```python
from build123d import *

# Parameters (mm, degrees)
SKETCH_1_R      = 2.08
SKETCH_1_R_2    = 8.75
SKETCH_1_R_3    = 1.5
EXTRUDE_2_DEPTH = 2


with BuildPart() as part:
    # 草图1 → 凸台-拉伸2 (new body)
    with BuildSketch(Plane.XY):
        with BuildLine():
            Line((25.488968202, 12.5), (30, 12.5))
            Line((30, 12.5), (30, 15.5))
            Line((30, 15.5), (37, 15.5))
            Line((37, 15.5), (37, 12.5))
            Line((37, 12.5), (41, 12.5))
            Line((41, 12.5), (41, 9.25))
            Line((41, 9.25), (44, 9.25))
            Line((44, 9.25), (44, 4.25))
            Line((44, 4.25), (41, 4.25))
            Line((41, 4.25), (41, 1.5))
            Line((41, 1.5), (38.5, 1.5))
            Line((38.5, 1.5), (38.5, 3))
            Line((38.5, 3), (35.9, 3))
            Line((35.9, 3), (35.9, 1.5))
            Line((35.9, 1.5), (32.9, 1.5))
            Line((32.9, 1.5), (32.9, -1.5))
            Line((32.9, -1.5), (35.9, -1.5))
            Line((35.9, -1.5), (35.9, -3))
            Line((35.9, -3), (38.5, -3))
            Line((38.5, -3), (38.5, -1.5))
            Line((38.5, -1.5), (41, -1.5))
            Line((41, -1.5), (41, -4.25))
            Line((41, -4.25), (44, -4.25))
            Line((44, -4.25), (44, -9.25))
            Line((44, -9.25), (41, -9.25))
            Line((41, -9.25), (41, -12.5))
            Line((41, -12.5), (37, -12.5))
            Line((37, -12.5), (37, -15.5))
            Line((37, -15.5), (30, -15.5))
            Line((30, -15.5), (30, -12.5))
            ThreePointArc((30, -12.5), (28.87224205, -11.37224205), (27.744484101, -12.5))
            Line((27.744484101, -12.5), (25.488968202, -12.5))
            ThreePointArc((25.488968202, -12.5), (0, -23.05787632), (-25.488968202, -12.5))
            Line((-25.488968202, -12.5), (-30, -12.5))
            Line((-30, -12.5), (-30, -15.5))
            Line((-30, -15.5), (-37, -15.5))
            Line((-37, -15.5), (-37, -12.5))
            Line((-37, -12.5), (-41, -12.5))
            Line((-41, -12.5), (-41, -9.25))
            Line((-41, -9.25), (-44, -9.25))
            Line((-44, -9.25), (-44, -4.25))
            Line((-44, -4.25), (-41, -4.25))
            Line((-41, -4.25), (-41, -1.5))
            Line((-41, -1.5), (-38.5, -1.5))
            Line((-38.5, -1.5), (-38.5, -3))
            Line((-38.5, -3), (-35.9, -3))
            Line((-35.9, -3), (-35.9, -1.5))
            Line((-35.9, -1.5), (-32.9, -1.5))
            Line((-32.9, -1.5), (-32.9, 1.5))
            Line((-32.9, 1.5), (-35.9, 1.5))
            Line((-35.9, 1.5), (-35.9, 3))
            Line((-35.9, 3), (-38.5, 3))
            Line((-38.5, 3), (-38.5, 1.5))
            Line((-38.5, 1.5), (-41, 1.5))
            Line((-41, 1.5), (-41, 4.25))
            Line((-41, 4.25), (-44, 4.25))
            Line((-44, 4.25), (-44, 9.25))
            Line((-44, 9.25), (-41, 9.25))
            Line((-41, 9.25), (-41, 12.5))
            Line((-41, 12.5), (-37, 12.5))
            Line((-37, 12.5), (-37, 15.5))
            Line((-37, 15.5), (-30, 15.5))
            Line((-30, 15.5), (-30, 12.5))
            Line((-30, 12.5), (-25.488968202, 12.5))
            ThreePointArc((-25.488968202, 12.5), (0, 23.05787632), (25.488968202, 12.5))
        make_face()
        with Locations((0, 13.53)):
            Circle(SKETCH_1_R, mode=Mode.SUBTRACT)
        with Locations((11.717323713, -6.765)):
            Circle(SKETCH_1_R, mode=Mode.SUBTRACT)
        with Locations((-11.717323713, -6.765)):
            Circle(SKETCH_1_R, mode=Mode.SUBTRACT)
        Circle(SKETCH_1_R_2, mode=Mode.SUBTRACT)
        with Locations((-12.990381057, 7.5)):
            Circle(SKETCH_1_R_3, mode=Mode.SUBTRACT)
        with Locations((12.990381057, 7.5)):
            Circle(SKETCH_1_R_3, mode=Mode.SUBTRACT)
        with Locations((0, -15)):
            Circle(SKETCH_1_R_3, mode=Mode.SUBTRACT)
    extrude(amount=EXTRUDE_2_DEPTH)


solid = part.part
```
Input: part model. Units: mm. Frame: model coordinates. A direction names the side the tool comes from. Give positions to 0.01 mm unless a question says otherwise; leave off trailing zeros. Loops run counter-clockwise (first coordinate to the right, second up) from the corner with the lowest first, then second, coordinate; pieces in that order, holes last.
1) Section query C-C on x = 10.5. Return the cut outline in (y, z), and give its area (3 significant figures).
A:
outline: (-21.49, 0) - (-8.45, 0) - (-8.45, 2) - (-21.49, 2) - close; (-5.08, 0) - (21.49, 0) - (21.49, 2) - (-5.08, 2) - close
area: 79.2 mm2
2) Reachability of faces 4 (the flat face through (30, -14, 1)), 5 (the flat face through (-43, -4.25, 1)), 6 (the flat face through (39, -12.5, 1)), 7 (the flat face through (-33, -15.5, 1)), 8 (the flat face through (43, 4.25, 1)) from +Z, -Z, +X, -X, +Y, -Y: full face, straight path, thin tool, end or side. Return the list, or none.
A:
face 4: +Z, -Z, -Y
face 5: +Z, -Z, -X
face 6: +Z, -Z, +X, -Y
face 7: +Z, -Z, -X, -Y
face 8: +Z, -Z, +X
3) Section query A-A on x = 0. Return the cut outline in (y, z), and give its area (3 significant figures).
A:
outline: (-23.06, 0) - (-16.5, 0) - (-16.5, 2) - (-23.06, 2) - close; (-13.5, 0) - (-8.75, 0) - (-8.75, 2) - (-13.5, 2) - close; (8.75, 0) - (11.45, 0) - (11.45, 2) - (8.75, 2) - close; (15.61, 0) - (23.06, 0) - (23.06, 2) - (15.61, 2) - close
area: 42.9 mm2
4) Line query: L1, parallel to Y at x = 0, z = 1.55; L2, parallel to Y at x = 36.5, z = 1.5; L3, parallel to Y at x = -40, z = 1.55. Output: solid intervals per line, ascending.
A:
L1: y = -23.06 to -16.5, -13.5 to -8.75, 8.75 to 11.45, 15.61 to 23.06
L2: y = -15.5 to -3, 3 to 15.5
L3: y = -12.5 to -1.5, 1.5 to 12.5
5) Section query D-D on y = 13.53. Return the cut outline in (x, z).
A:
outline: (-37, 0) - (-30, 0) - (-30, 2) - (-37, 2) - close; (-24.42, 0) - (-2.08, 0) - (-2.08, 2) - (-24.42, 2) - close; (2.08, 0) - (24.42, 0) - (24.42, 2) - (2.08, 2) - close; (30, 0) - (37, 0) - (37, 2) - (30, 2) - close
6) Mould query, pull axis Y, two halves, no side actions, for faces 1 (the flat face through (38.5, -2, 1)), 2 (the flat face through (44, 7, 1)), 3 (the flat face through (28, 12.5, 1)). Classes: released by +Y, released by -Y, zero draft, split by the parting line, or undercut.
A:
face 1: undercut
face 2: zero draft
face 3: released by +Y
7) Section query B-B on y = 0. Return the cut outline in (x, z).
A:
outline: (-32.9, 0) - (-8.75, 0) - (-8.75, 2) - (-32.9, 2) - close; (8.75, 0) - (32.9, 0) - (32.9, 2) - (8.75, 2) - close
8) Contact query for flat-ended pins moving along their axis: pin 1 (1 mm diameter, centred on x = -42, z = 1, fed in from -Y); pin 2 (1 mm diameter, centred on x = 38.5, z = 1.5, fed in from -Y); pin 3 (5 mm diameter, centred on x = 0, y = -15, fed in from +Z); pin 4 (0.6 mm diameter, centred on x = 34.5, z = 0.5, fed in from +Y). Output: stop coordinate, or through.
A:
pin 1: stops at y = -9.25
pin 2: stops at y = -12.5
pin 3: stops at z = 2
pin 4: stops at y = 15.5
